Source: CAD feature listing. Evaluate the final solid. Frame: model axes, mm. A direction names the side the tool comes from. Give positions to 0.01 mm unless a question says otherwise; leave off trailing zeros. Order: outer loops, then holes, each group sorted by start corner. A loop starts at its lowest first (then second) coordinate and runs counter-clockwise, first axis right, second up. Notation, with made-up numbers: M -18,-21 L -14,-21 A24 ccw -14,13 Z; hole C 25.25,77 d9. An arc over 180 degrees is marked long. Answer in a Markdown table with one row per item. Add a question column.
(1) Section query D-D, the plane z = 58.5. Return loops of the section in (x, y).
(2) Pin query (flat end, axial travel): P1, Ø1.5, axis at x = 15, z = 151, coming from the +Y side; P2, Ø6, axis at x = 19, z = -7.5, coming from the +Y side; P3, Ø6.5, axis at x = -21.5, y = -16, coming from the +Z side. Return the tip coordinate at first contact, or that it passes through.
(3) Set-up query: faces 1 (the face through (-13.887, -10.648, 56.723)), 2 (the face through (27, 7, -345.5)), 3 (the face through (29.97, 1.32, -246.9)). Return all of +Z, -Z, +X, -X, +Y, -Y with unobstructed straight access to the full face (end or side cutting, diameter ignored); none if empty.
(4) Material intervals for line 1 along X through (y, z) = (5.5, 330); line 2 along Y through (x, z) = (-9, 340); line 3 along Z through (x, y) = (-15, 5), sorted ascending.
(5) Section query C-C, the plane z = 294. Return loops of the section in (x, y).
(6) Section query A-A, the plane x = 0. Return loops of the section in (y, z).
Autodesk Inventor part; units mm, degrees
ref_plane "YZ Plane" through (0, 0, 0) normal (1, 0, 0) x (0, 1, 0)
ref_plane "XZ Plane" through (0, 0, 0) normal (0, 1, 0) x (-1, 0, 0)
ref_plane "XY Plane" through (0, 0, 0) normal (0, 0, 1) x (1, 0, 0)
sketch "Sketch1" plane through (0, 0, 0) normal (0, 0, 1) x (1, 0, 0)
  circle A0 centre (0, 0) radius 17.5
  dimension "d0" = 35
extrude "Extrusion1" add sketch "Sketch1" along normal mid plane 725
sketch "Sketch3" plane through (0, 0, 362.5) normal (0, 0, 1) x (1, 0, 0)
  circle A0 centre (0, 0) radius 15
  circle A1 centre (0, 0) radius 17.5
  dimension "d6" = 30
extrude "Extrusion3" cut sketch "Sketch3" against normal blind 114
sketch "Sketch4" plane through (0, 0, 362.5) normal (0, 0, 1) x (1, 0, 0)
  circle A0 centre (0, 0) radius 14
  circle A1 centre (0, 0) radius 15
  dimension "d9" = 28
extrude "Extrusion4" cut sketch "Sketch4" against normal blind 22
thread "Thread1"
sketch "Sketch5" plane through (0, 0, 362.5) normal (0, 0, 1) x (1, 0, 0)
  circle A0 centre (0, 0) radius 14
extrude "Extrusion5" add sketch "Sketch5" along normal blind 10
fillet "Fillet1" radius 2 1 edges at (-14, 0, 372.5)
sketch "Sketch6" plane through (0, 0, 248.5) normal (0, 0, 1) x (1, 0, 0)
  line L0 (11.1074, -10.3393) -> (14.156, -14.3025)
  line L1 (7.1443, -13.3879) -> (11.1074, -10.3393)
  line L2 (7.1443, -13.3879) -> (10.1929, -17.351)
  line L3 (10.1929, -17.351) -> (14.156, -14.3025)
  point P0 (0, 0)
extrude "Extrusion6" cut sketch "Sketch6" along normal blind 55
sketch "Sketch7" plane through (0, 0, -362.5) normal (0, 0, -1) x (-1, 0, 0)
  circle A0 centre (0, 0) radius 17.5
extrude "Extrusion7" cut sketch "Sketch7" against normal blind 17
sketch "Sketch8" plane through (0, 0, -345.5) normal (0, 0, -1) x (-1, 0, 0)
  circle A0 centre (0, 0) radius 30
  dimension "d21" = 60
extrude "Extrusion8" add sketch "Sketch8" against normal blind 200
fillet "Fillet2" radius 5 1 edges at (-17.5, 0, -145.5)
sketch "Sketch9" plane through (0, 0, -345.5) normal (0, 0, -1) x (-1, 0, 0)
  circle A0 centre (0, 0) radius 17.5
  circle A1 centre (0, 0) radius 27.5
  dimension "d25" = 55
extrude "Extrusion9" add sketch "Sketch9" along normal blind 50 contours A0 | A1
sketch "Sketch10" plane through (0, 0, -345.5) normal (0, 0, -1) x (-1, 0, 0)
  line L0 (59.3657, -110.0033) -> (360.8409, -346.1125)
  arc A0 (360.8409, -346.1125) -> (422.4996, -267.3838) centre (0, 0) ccw
  line L1 (422.4996, -267.3838) -> (121.0244, -31.2746)
  arc A1 (121.0244, -31.2746) -> (65.5828, 106.4138) centre (0, 0) ccw
  line L2 (65.5828, 106.4138) -> (119.3218, 485.5536)
  arc A2 (119.3218, 485.5536) -> (20.3114, 499.5873) centre (0, 0) ccw
  line L3 (20.3114, 499.5873) -> (-33.4276, 120.4475)
  arc A3 (-33.4276, 120.4475) -> (-124.9485, 3.5894) centre (0, 0) ccw
  line L4 (-124.9485, 3.5894) -> (-480.1627, -139.4411)
  arc A4 (-480.1627, -139.4411) -> (-442.811, -232.2034) centre (0, 0) ccw
  line L5 (-442.811, -232.2034) -> (-87.5968, -89.1729)
  arc A5 (-87.5968, -89.1729) -> (59.3657, -110.0033) centre (0, 0) ccw
  line L6 (25.8741, -15.1833) -> (28.4468, -17.1982)
  line L7 (28.4468, -17.1982) -> (23.5141, -23.4965)
  line L8 (23.5141, -23.4965) -> (20.9414, -21.4816)
  arc A6 (25.8741, -15.1833) -> (20.9414, -21.4816) centre (0, 0) ccw
  line L9 (23.5141, -23.4965) -> (28.4468, -17.1982)
  line L10 (28.4468, -17.1982) -> (22.9358, -12.8821)
  line L11 (22.9358, -12.8821) -> (18.0031, -19.1804)
  line L12 (18.0031, -19.1804) -> (23.5141, -23.4965)
  point P0 (0, 0)
  dimension "d28" = 7
  dimension "d31" = 8
extrude "Extrusion10" cut sketch "Sketch10" against normal blind 100 contours L6 L7 L8 L12 L11 L10
thread "Thread2"
fillet "Fillet3" radius 5 1 edges at (27.5, 0, -395.5)
properties part number "Lower Shaft"
Values follow:
| question | item | result |
|---|---|---|
| 1 | outline | C 0,0 d35 |
| 2 | P1 | stops at y = 10.16 |
| 2 | P2 | stops at y = 7.09 |
| 2 | P3 | stops at z = -145.5 |
| 3 | face 1 | +Z |
| 3 | face 2 | -Z |
| 3 | face 3 | +Z, -Z |
| 4 | line 1 | x = -13.96 to 13.96 |
| 4 | line 2 | y = -12 to 12 |
| 4 | line 3 | z = -395.5 to 248.5 |
| 5 | outline | M 8.34,-12.47 L 9.91,-11.26 A15 ccw long Z |
| 6 | outline | M -30,-345.5 L -27.5,-345.5 L -27.5,-390.5 A5 ccw -22.5,-395.5 L 22.5,-395.5 A5 ccw 27.5,-390.5 L 27.5,-345.5 L 30,-345.5 L 30,-145.5 L 22.5,-145.5 A5 cw 17.5,-140.5 L 17.5,248.5 L 15,248.5 L 15,340.5 L 14,340.5 L 14,370.5 A2 ccw 12,372.5 L -12,372.5 A2 ccw -14,370.5 L -14,340.5 L -15,340.5 L -15,248.5 L -17.5,248.5 L -17.5,-140.5 A5 cw -22.5,-145.5 L -30,-145.5 Z |
